```python
from build123d import *

# Parameters (mm, degrees)
F0_W     = 100
F0_H     = 150
F1_DEPTH = 20
F2_R     = 5
F3_D     = 5
F3_DEPTH = 12
F3_TIP   = 1.5021515476
F4_W     = 10
F4_H     = 150
F5_DEPTH = 5
F6_F1_R  = 4.9999
F6_F2_R  = 5


# Not quite as in the source:
# - a fillet or chamfer is up to 0.001 mm smaller than in the source, because OpenCascade refuses the exact size


with BuildPart() as f1:
    # F0 (on Top) → F1 (new body)
    with BuildSketch(Plane.XY):
        Rectangle(F0_W, F0_H)
    extrude(amount=F1_DEPTH)

    # F2
    f2_edges = [f1.edges().sort_by_distance(p)[0] for p in [
        (-50, 75, 10),
        (50, 75, 10),
        (0, -75, 20),
        (50, 0, 20),
        (0, 75, 20),
        (-50, 0, 20),
        (50, -75, 10),
        (-50, -75, 10),
    ]]
    fillet(f2_edges, radius=F2_R)

    # F3
    with Locations(Plane(origin=(0, 0, 0), x_dir=(1, 0, 0), z_dir=(0, 0, -1))):
        with Locations((40, -65), (-40, -65), (40, 65), (-40, 65)):
            Hole(F3_D / 2, depth=F3_DEPTH)
            with Locations((0, 0, -(F3_DEPTH + F3_TIP / 2))):  # 118° drill point
                Cone(0, F3_D / 2, F3_TIP, mode=Mode.SUBTRACT)

    # F4 (on face) → F5 (cut)
    with BuildSketch(Plane.XY):
        Rectangle(F4_W, F4_H)
    extrude(amount=F5_DEPTH, mode=Mode.SUBTRACT)

    # F6: fillet of radius 5 on 4 edges, made by hand

    # F6_f1 (radius 5 in the source; OpenCascade refuses exactly that, so slightly less here)
    f6_f1_edges = [f1.edges().sort_by_distance(p)[0] for p in [
        (5, 0, 5),
        (-5, 0, 5),
    ]]
    fillet(f6_f1_edges, radius=F6_F1_R)

    # F6_f2
    f6_f2_edges = [f1.edges().sort_by_distance(p)[0] for p in [
        (5, -75, 5e-05),
        (-5, 75, 5e-05),
        (-3.5355631953, 75, 3.5355631953),
        (3.5355631953, -75, 3.5355631953),
    ]]
    fillet(f6_f2_edges, radius=F6_F2_R)


solid = f1.part
```
Part model, mm, in its own coordinate system. A direction names the side the tool comes from. Give positions to 0.01 mm unless a question says otherwise; leave off trailing zeros. Use a Markdown table: item, result. Add a question column.
(1) Mould opens along Y. For faces 1 (the face through (37.69, 65.96, 6.08)), 2 (the face through (50, -1, 7)), 3 (the face through (-1, 75, 11)), 4 (the face through (40.23, 64.63, 13.24)) say: +Y half, -Y half, draft (parallel to the pull), parting line (faces both ways), or undercut.
(2) Probe line 1 along Y through (x, z) = (-40, 9.5); line 2 along X through (y, z) = (-65, 6.5); line 3 along X through (y, z) = (-66, 5.75). List the from-to ranges inside material, lowest first. Write a range as [from, to].
(3) 3-axis set-ups, long thin cutter, end or side, ignore diameter. For faces 5 (the face through (-42.31, 65.96, 6.08)), 6 (the face through (3, 1, 4)), 7 (the face through (-1, -75, 11)): which of +Z, -Z, +X, -X, +Y, -Y reach the whole face in a straight line?
Answer key:
| question | item | result |
|---|---|---|
| 1 | face 1 | undercut |
| 1 | face 2 | draft |
| 1 | face 3 | +Y half |
| 1 | face 4 | undercut |
| 2 | line 1 | [-75, -67.5], [-62.5, 62.5], [67.5, 75] |
| 2 | line 2 | [-50, -42.5], [-37.5, 37.5], [42.5, 50] |
| 2 | line 3 | [-50, -42.29], [-37.71, 37.71], [42.29, 50] |
| 3 | face 5 | -Z |
| 3 | face 6 | -Z, +Y, -Y |
| 3 | face 7 | +Z, -Z, +X, -X, -Y |
